Check sheet for the drawn part. Datum: minimum x, y, z corner. Units: mm. A direction names the side the tool comes from. Round coordinates to 2 decimals unless told otherwise and drop trailing zeros. Write each loop counter-clockwise with the first axis right and the second up, starting at its lowest first coordinate (ties: lowest second). Pieces come first, ordered by that corner, then holes. Notation, with made-up numbers: (42, -39.5) -> (94, -39.5) arc R32 ccw to (94, -3.5) -> close; hole circle Ø1 at (-20, -23.75). An arc over 180 degrees is marked (long way). Use CSV: the item, a comma, the result in double quotes.
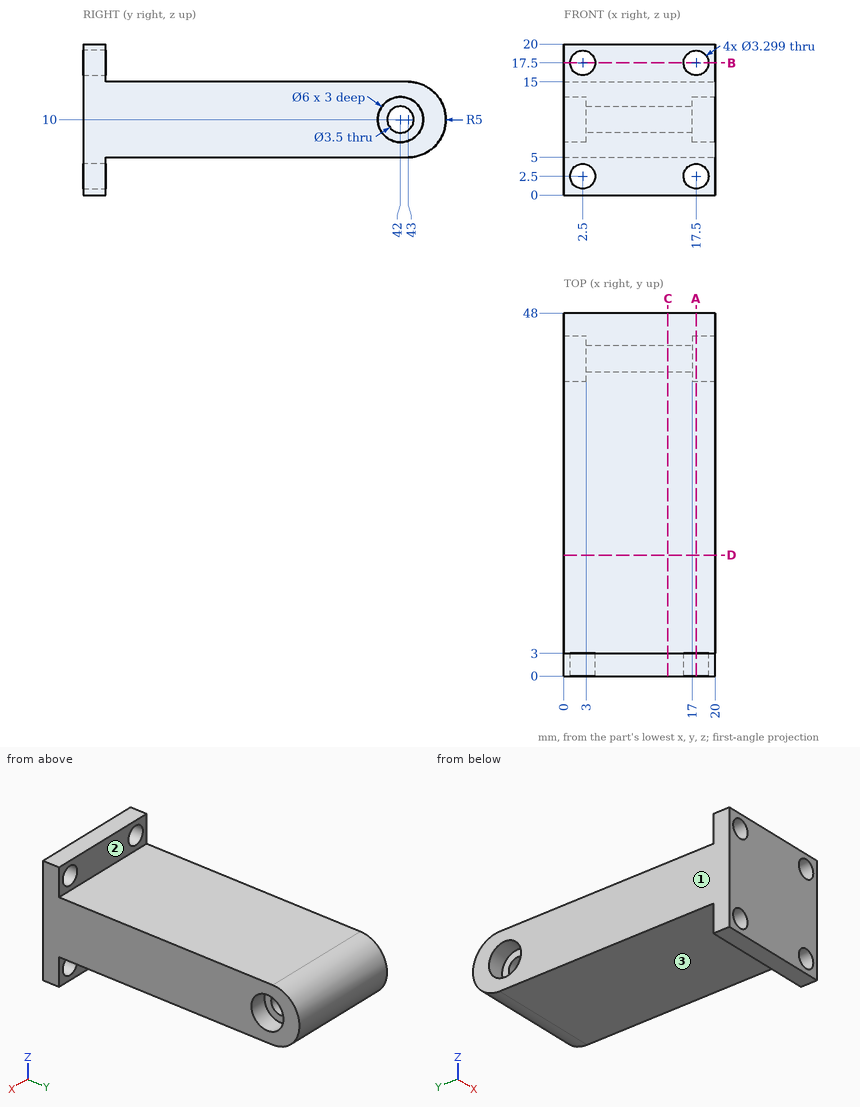
Q1. Section check D-D (y = 16). Record the cut outline in (x, z).
Filled in:
outline,"(0, 5) -> (20, 5) -> (20, 15) -> (0, 15) -> close"
Q2. Access from +Z, -Z, +X, -X, +Y, -Y to the whole of each face (thin tool, end or side, straight path). Record for the marked faces 1, 2 and 3.
Filled in:
face 1,"+Z, -Z, -X, +Y, -Y"
face 2,"+Z, +X, -X, +Y"
face 3,"-Z, +X, -X, +Y"
Q3. Section check B-B (z = 17.5). Record the cut outline in (x, y), plus the area to 3 significant figures.
Filled in:
outline,"(0, 0) -> (0.85, 0) -> (0.85, 3) -> (0, 3) -> close; (4.15, 0) -> (15.85, 0) -> (15.85, 3) -> (4.15, 3) -> close; (19.15, 0) -> (20, 0) -> (20, 3) -> (19.15, 3) -> close"
area,"40.2 mm²"
Q4. Section check A-A (x = 17.5). Record the cut outline in (y, z), plus the area to 3 significant figures.
Filled in:
outline,"(0, 0) -> (3, 0) -> (3, 0.85) -> (0, 0.85) -> close; (0, 4.15) -> (3, 4.15) -> (3, 5) -> (43, 5) arc R5 ccw to (43, 15) -> (3, 15) -> (3, 15.85) -> (0, 15.85) -> close; (0, 19.15) -> (3, 19.15) -> (3, 20) -> (0, 20) -> close; hole circle Ø6 at (42, 10)"
area,"451 mm²"
Q5. Go/stop test with flat-tipped pins: P1, Ø10, axis at x = 16.5, y = 32, coming from the +Z side; P2, Ø1, axis at x = 11.5, z = 11.5, coming from the +Y side; P3, Ø5, axis at y = 42, z = 10, coming from the -X side; P4, Ø2, axis at x = 2.5, z = 17.5, coming from the -Y side. Record where each tip stops, or that it passes through.
Filled in:
P1,"z = 15"
P2,"y = 47.9"
P3,"x = 3"
P4,"through"
Q6. Material ranges on L1, parallel to X at y = 1.25, z = 17.5; L2, parallel to Y at x = 2.2, z = 10; L3, parallel to Z at x = 1.2, y = 42, recorded low to high.
Filled in:
L1,"0 to 0.85, 4.15 to 15.85, 19.15 to 20"
L2,"0 to 39, 45 to 48"
L3,"5 to 7, 13 to 15"
Q7. Section check C-C (x = 13.75). Record the cut outline in (y, z).
Filled in:
outline,"(0, 0) -> (3, 0) -> (3, 5) -> (43, 5) arc R5 ccw to (43, 15) -> (3, 15) -> (3, 20) -> (0, 20) -> close; hole circle Ø3.5 at (42, 10)"
